Geometry check sheet. Reference: the model listing, model coordinates, mm. Face numbers are marked on the shaded views. Give positions to 0.01 mm unless a question says otherwise; leave off trailing zeros. Write each loop counter-clockwise with the first axis right and the second up, starting at its lowest first coordinate (ties: lowest second). Pieces come first, ordered by that corner, then holes. Notation, with made-up numbers: (-10, -17) -> (28, -17) arc R34 ccw to (28, 14) -> close; hole circle Ø3 at (-21, -37). An arc over 180 degrees is marked (long way). Use a Markdown table: item, result. Add a question column.
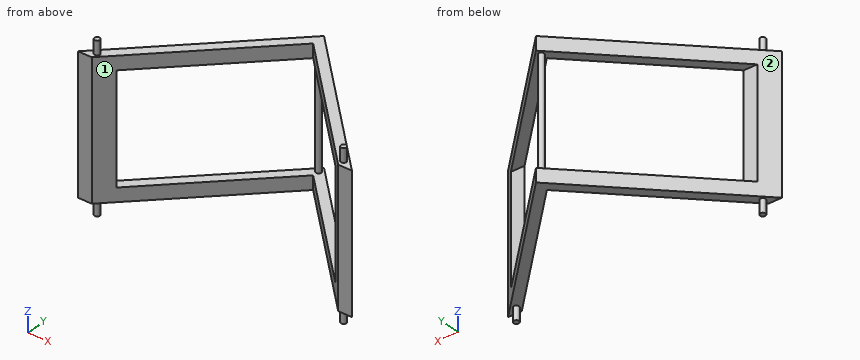
from build123d import *

# Parameters (mm, degrees)
BOSS_EXTRUDE2_DEPTH     = 250
CUT_EXTRUDE1_DEPTH      = 751
CUT_EXTRUDE1_DEPTH_BACK = 751
SKETCH4_W               = 400
SKETCH4_H               = 450
BOSS_EXTRUDE3_REACH     = 840.153
SKETCH6_R               = 10
SKETCH7_R               = 10
BOSS_EXTRUDE4_DEPTH     = 50
MIRROR2_COPY_1_SKETCH_R = 10
MIRROR2_COPY_1_DEPTH    = 50


with BuildPart() as part:
    # Sketch2 → Boss-Extrude2 (new, symmetric)
    with BuildSketch(Plane.XY):
        Polygon((-500, 0), (0, 500), (500, 0), (450, 0), (0, 450), (-450, 0), align=None)
    extrude(amount=BOSS_EXTRUDE2_DEPTH, both=True)

    # Sketch4 → Cut-Extrude1 (cut, two sides: drawn at the far end of the back side and taken through both)
    with BuildSketch(Plane(origin=(0, 0, 0), x_dir=(0, 0, -1), z_dir=(1, 0, 0)).offset(-CUT_EXTRUDE1_DEPTH_BACK)):
        with Locations((0, 275)):
            Rectangle(SKETCH4_W, SKETCH4_H)
    extrude(amount=CUT_EXTRUDE1_DEPTH + CUT_EXTRUDE1_DEPTH_BACK, mode=Mode.SUBTRACT)

    # Sketch6 → Boss-Extrude3 (add, up to next)
    with BuildSketch(Plane(origin=(0, 0, 200), x_dir=(-1, 0, 0), z_dir=(0, 0, -1)), mode=Mode.PRIVATE) as boss_extrude3_sk1:
        with Locations(Location((0, 475, 0), (0, 0, 270))):
            Circle(SKETCH6_R)
    boss_extrude3_tool1 = extrude(boss_extrude3_sk1.sketch, amount=BOSS_EXTRUDE3_REACH, mode=Mode.PRIVATE) - part.part
    add(boss_extrude3_tool1.solids().sort_by_distance((0, 475, 200))[0])

    # Sketch7 → Boss-Extrude4 (add)
    with BuildSketch(Plane.XY.offset(250)):
        with Locations(Location((450, 25, 0), (0, 0, 180))):
            Circle(SKETCH7_R)
    boss_extrude4 = extrude(amount=BOSS_EXTRUDE4_DEPTH)

    # Mirror1: Boss-Extrude4 across plane
    add(boss_extrude4.mirror(Plane.XY))

    # Mirror2: Boss-Extrude4 across plane
    add(boss_extrude4.mirror(Plane(origin=(0, 0, 0), x_dir=(0, 0, 1), z_dir=(1, 0, 0))))

    # Mirror2 copy 1 sketch → Mirror2 copy 1 (add)
    with BuildSketch(Plane(origin=(0, 0, -250), x_dir=(-1, 0, 0), z_dir=(0, 0, -1))):
        with Locations(Location((450, 25, 0), (0, 0, 180))):
            Circle(MIRROR2_COPY_1_SKETCH_R)
    extrude(amount=MIRROR2_COPY_1_DEPTH)


solid = part.part
1) Draft check along X on the marked faces 1 and 2. Enter one of: +X half, -X half, draft (parallel to the pull), parting line (faces both ways), or undercut.
2) Material ranges on probe 1 along Z at (x, y) = (-437, 51); probe 2 along X at (y, z) = (44.5, 177.5); probe 3 along X at (y, z) = (319, 201), recorded low to high. Write a range as [from, to].
3) Sectioned sample at A-A, the plane x = 313. Enter the section's corners in (y, z).
4) Sectioned sample at B-B, the plane y = 400. Enter the section's corners in (x, z), and give its area (3 significant figures).
5) Sectioned sample at C-C, the plane z = -15.5. Enter the section's corners in (x, y).
6) Gauge pin test, flat ends, axial feed: P1, Ø8, axis at x = -11, z = -3.5, coming from the -Y side; P2, Ø12, axis at y = 384.5, z = -206.5, coming from the -X side; P3, Ø15, axis at x = 422.5, z = -57.5, coming from the +Y side. Record the tip position at first contact, or that the pin passes through.
Check values:
| question | item | result |
|---|---|---|
| 1 | face 1 | undercut |
| 1 | face 2 | -X half |
| 2 | probe 1 | [-250, -200], [200, 250] |
| 2 | probe 2 | [-455.5, -405.5], [405.5, 455.5] |
| 2 | probe 3 | [-181, -131], [131, 181] |
| 3 | outline | (137, -250) -> (187, -250) -> (187, -200) -> (137, -200) -> close; (137, 200) -> (187, 200) -> (187, 250) -> (137, 250) -> close |
| 4 | outline | (-100, -250) -> (-50, -250) -> (-50, -200) -> (-100, -200) -> close; (-100, 200) -> (-50, 200) -> (-50, 250) -> (-100, 250) -> close; (50, -250) -> (100, -250) -> (100, -200) -> (50, -200) -> close; (50, 200) -> (100, 200) -> (100, 250) -> (50, 250) -> close |
| 4 | area | 10,000 mm² |
| 5 | outline | (-500, 0) -> (-450, 0) -> (-400, 50) -> (-450, 50) -> close; circle Ø20 at (0, 475); (400, 50) -> (450, 0) -> (500, 0) -> (450, 50) -> close |
| 6 | P1 | y = 467.86 |
| 6 | P2 | x = -121.5 |
| 6 | P3 | y = 50 |
